```python
from build123d import *

# Parameters (mm, degrees)
SKETCH1_W           = 63.5
SKETCH1_H           = 6.35
BOSS_EXTRUDE1_DEPTH = 53.34
BOSS_EXTRUDE2_DEPTH = 6.35
CUT_EXTRUDE1_REACH  = 94.454
SKETCH11_R          = 4.445
FILLET1_R           = 2.54
CUT_EXTRUDE2_REACH  = 94.454
SKETCH19_R          = 1.778


with BuildPart() as part:
    # Sketch1 → Boss-Extrude1 (new body)
    with BuildSketch(Plane(origin=(0, 0, 0), x_dir=(0, 0, -1), z_dir=(1, 0, 0))):
        with Locations((31.75, 3.175)):
            Rectangle(SKETCH1_W, SKETCH1_H)
    extrude(amount=-BOSS_EXTRUDE1_DEPTH)

    # Sketch2 → Boss-Extrude2 (add)
    with BuildSketch(Plane(origin=(0, 0, 0), x_dir=(0, 0, -1), z_dir=(1, 0, 0))):
        Polygon((0, 6.35), (0, 26.67), (12.7, 40.869031657), (50.8, 40.869031657), (63.5, 26.67), (63.5, 6.35), align=None)
    boss_extrude2 = extrude(amount=-BOSS_EXTRUDE2_DEPTH)

    # Sketch11 → Cut-Extrude1 (cut, up to next)
    with BuildSketch(Plane(origin=(0, 0, 0), x_dir=(0, 0, -1), z_dir=(1, 0, 0)), mode=Mode.PRIVATE) as cut_extrude1_sk1:
        with Locations((19.05, 26.391031657)):
            Circle(SKETCH11_R)
    cut_extrude1_tool1 = extrude(cut_extrude1_sk1.sketch, amount=-CUT_EXTRUDE1_REACH, mode=Mode.PRIVATE) & part.part
    # Sketch11 → Cut-Extrude1 (cut, up to next)
    with BuildSketch(Plane(origin=(0, 0, 0), x_dir=(0, 0, -1), z_dir=(1, 0, 0)), mode=Mode.PRIVATE) as cut_extrude1_sk2:
        with Locations((44.45, 26.391031657)):
            Circle(SKETCH11_R)
    cut_extrude1_tool2 = extrude(cut_extrude1_sk2.sketch, amount=-CUT_EXTRUDE1_REACH, mode=Mode.PRIVATE) & part.part
    cut_extrude1_1 = cut_extrude1_tool1.solids().sort_by_distance((0, 26.391032, -19.05))[0]
    add(cut_extrude1_1, mode=Mode.SUBTRACT)
    cut_extrude1_2 = cut_extrude1_tool2.solids().sort_by_distance((0, 26.391032, -44.45))[0]
    add(cut_extrude1_2, mode=Mode.SUBTRACT)
    cut_extrude1 = cut_extrude1_1 + cut_extrude1_2  # Cut-Extrude1 as one shape, for the pattern or mirror that repeats it

    # Fillet1
    fillet1_edges = [part.edges().sort_by_distance(p)[0] for p in [
        (0, 0, -31.75),
        (-53.34, 0, -31.75),
        (-26.67, 0, -63.5),
        (-26.67, 0, 0),
    ]]
    fillet(fillet1_edges, radius=FILLET1_R)

    # Sketch19 → Cut-Extrude2 (cut, up to next)
    with BuildSketch(Plane.XZ, mode=Mode.PRIVATE) as cut_extrude2_sk1:
        with Locations(Location((-10.795, -50.8, 0), (0, 0, 270))):
            Circle(SKETCH19_R)
    cut_extrude2_tool1 = extrude(cut_extrude2_sk1.sketch, amount=-CUT_EXTRUDE2_REACH, mode=Mode.PRIVATE) & part.part
    # Sketch19 → Cut-Extrude2 (cut, up to next)
    with BuildSketch(Plane.XZ, mode=Mode.PRIVATE) as cut_extrude2_sk2:
        with Locations(Location((-42.545, -50.8, 0), (0, 0, 270))):
            Circle(SKETCH19_R)
    cut_extrude2_tool2 = extrude(cut_extrude2_sk2.sketch, amount=-CUT_EXTRUDE2_REACH, mode=Mode.PRIVATE) & part.part
    # Sketch19 → Cut-Extrude2 (cut, up to next)
    with BuildSketch(Plane.XZ, mode=Mode.PRIVATE) as cut_extrude2_sk3:
        with Locations(Location((-42.545, -12.7, 0), (0, 0, 270))):
            Circle(SKETCH19_R)
    cut_extrude2_tool3 = extrude(cut_extrude2_sk3.sketch, amount=-CUT_EXTRUDE2_REACH, mode=Mode.PRIVATE) & part.part
    # Sketch19 → Cut-Extrude2 (cut, up to next)
    with BuildSketch(Plane.XZ, mode=Mode.PRIVATE) as cut_extrude2_sk4:
        with Locations(Location((-10.795, -12.7, 0), (0, 0, 270))):
            Circle(SKETCH19_R)
    cut_extrude2_tool4 = extrude(cut_extrude2_sk4.sketch, amount=-CUT_EXTRUDE2_REACH, mode=Mode.PRIVATE) & part.part
    add(cut_extrude2_tool1.solids().sort_by_distance((-10.795, 0, -50.8))[0], mode=Mode.SUBTRACT)
    add(cut_extrude2_tool2.solids().sort_by_distance((-42.545, 0, -50.8))[0], mode=Mode.SUBTRACT)
    add(cut_extrude2_tool3.solids().sort_by_distance((-42.545, 0, -12.7))[0], mode=Mode.SUBTRACT)
    add(cut_extrude2_tool4.solids().sort_by_distance((-10.795, 0, -12.7))[0], mode=Mode.SUBTRACT)

    # Mirror1: Boss-Extrude2, Cut-Extrude1 across plane
    add(boss_extrude2.mirror(Plane(origin=(-26.67, 0, 0), x_dir=(0, 0, 1), z_dir=(1, 0, 0))))
    add(cut_extrude1.mirror(Plane(origin=(-26.67, 0, 0), x_dir=(0, 0, 1), z_dir=(1, 0, 0))), mode=Mode.SUBTRACT)


solid = part.part
```
Check sheet for the modelled part. Datum: model origin and axes. Units: mm. A direction names the side the tool comes from. Give positions to 0.01 mm unless a question says otherwise; leave off trailing zeros. Write each loop counter-clockwise with the first axis right and the second up, starting at its lowest first coordinate (ties: lowest second). Pieces come first, ordered by that corner, then holes.
Item 1: Draft check along Y on faces 1 (the face through (-26, 6.35, -31)), 2 (the face through (-42.467, 3.131, -49.024)), 3 (the face through (-50.21, 27.73, -23.29)). Enter one of: released by +Y, released by -Y, zero draft, split by the parting line, or undercut.
Item 2: Cross-section at D-D (x = -19). Enter the section's corners in (y, z), and give its area (3 significant figures).
Item 3: Scan lines: L1, parallel to X at y = 5, z = -50.8; L2, parallel to Z at x = -6, y = 26.5; L3, parallel to X at y = 31, z = -36. Record each from-to range of solid material in increasing order.
Item 4: Cross-section at C-C (z = -25.5). Enter the section's corners in (x, y), and give its area (3 significant figures).
Item 5: Access from +Z, -Z, +X, -X, +Y, -Y to the whole of each face (thin tool, end or side, straight path). Record for faces 4 (the face through (-46.99, 24, -32)), 5 (the face through (-26, 0, -31)).
Item 6: Gauge pin test, flat end, axial feed: pin 1 (12 mm diameter, centred on x = -37, z = -33, fed in from +Y). Record the tip position at first contact, or that the pin passes through.
Item 7: Cross-section at A-A (z = -44.45). Enter the section's corners in (x, y), and give its area (3 significant figures).
Item 8: Cross-section at B-B (y = 35.5). Enter the section's corners in (x, z), and give its area (3 significant figures).
Report:
1. face 1: released by +Y
1. face 2: zero draft
1. face 3: undercut
2. outline: (0, -60.96) arc R2.54 ccw to (2.54, -63.5) - (6.35, -63.5) - (6.35, 0) - (2.54, 0) arc R2.54 ccw to (0, -2.54) - close
2. area: 400 mm2
3. L1: x = -53.34 to -44.32, -40.77 to -12.57, -9.02 to 0
3. L2: z = -63.5 to -48.89, -40.01 to -23.49, -14.61 to 0
3. L3: x = -53.34 to -46.99, -6.35 to 0
4. outline: (-53.34, 2.54) arc R2.54 ccw to (-50.8, 0) - (-2.54, 0) arc R2.54 ccw to (0, 2.54) - (0, 40.87) - (-6.35, 40.87) - (-6.35, 6.35) - (-46.99, 6.35) - (-46.99, 40.87) - (-53.34, 40.87) - close
4. area: 774 mm2
5. face 4: +Z, -Z, +Y
5. face 5: +Z, -Z, +X, -X, -Y
6. pin 1: stops at y = 6.35
7. outline: (-53.34, 2.54) arc R2.54 ccw to (-50.8, 0) - (-2.54, 0) arc R2.54 ccw to (0, 2.54) - (0, 21.95) - (-6.35, 21.95) - (-6.35, 6.35) - (-46.99, 6.35) - (-46.99, 21.95) - (-53.34, 21.95) - close; (-53.34, 30.84) - (-46.99, 30.84) - (-46.99, 40.87) - (-53.34, 40.87) - close; (-6.35, 30.84) - (0, 30.84) - (0, 40.87) - (-6.35, 40.87) - close
7. area: 661 mm2
8. outline: (-53.34, -55.6) - (-46.99, -55.6) - (-46.99, -7.9) - (-53.34, -7.9) - close; (-6.35, -55.6) - (0, -55.6) - (0, -7.9) - (-6.35, -7.9) - close
8. area: 606 mm2
